The model under review builds one solid part; all positions refer to its coordinate system, in mm. A direction names the side the tool comes from. Round coordinates to 2 decimals unless told otherwise and drop trailing zeros. Order: outer loops, then holes, each group sorted by start corner. A loop starts at its lowest first (then second) coordinate and runs counter-clockwise, first axis right, second up. Notation, with made-up numbers: M 48,-11 L 100,-11 A20 ccw 100,27 Z; hole C 6.5,-12 d4. An arc over 180 degrees is marked long. Answer as a JSON object with one key per item and string values. Group by question number.
1) For faces 1 (the flat face through (30.94, -1, 2)), 2 (the flat face through (2, 11.298, 2)), 3 (the cylindrical face through (54.597, 7.345, 1.551)), 4 (the flat face through (25.06, 46, 2)), list the 3-axis set-ups (+Z, -Z, +X, -X, +Y, -Y) from which the entire face can be reached by the end or side of a thin tool; tool diameter is ignored.
2) Consider section A-A, the plane x = 2.5. Write out the cut boundary in (y, z), then the cut area to 3 significant figures.
3) To check wall thickness, follow line 1 (Y direction, x = 53.5, z = 0.85); line 2 (Y direction, x = 2.5, z = 2.3); line 3 (X direction, y = 26.5, z = 0.95). State the ranges of each line that lie inside material, in increasing order.
4) Consider section B-B, the plane z = 1.5. Write out the cut boundary in (x, y).
5) Consider section D-D, the plane y = 20.5. Write out the cut boundary in (x, z).
6) Consider section C-C, the plane x = 53.5. Write out the cut boundary in (y, z).
7) Insertion check: pin 1 Ø0.9 at (x, z) = (27, 1.5) entering from -Y. The pin has a flat end and moves straight along its axis. Give the tip position at first contact, or say it passes through.
8) The part is to be moulded in two halves that separate along X. For faces 5 (the flat face through (0, 41, 2)), 6 (the flat face through (13, 48, 2)), 7 (the cylindrical face through (2.251, 36.377, 1.551)), say which applies: +X half, -X half, draft (parallel to the pull), parting line (faces both ways), or undercut.
```python
from build123d import *

# Parameters (mm, degrees)
BOSS_EXTRUDE1_DEPTH = 3.06
SKETCH2_R           = 1.15
SKETCH2_W           = 4
SKETCH2_H           = 22.201866978
CUT_EXTRUDE1_DEPTH  = 74.819804931


with BuildPart() as part:
    # Sketch1 → Boss-Extrude1 (new body)
    with BuildSketch(Plane.XY):
        Polygon((25.06, 0), (30.94, 0), (30.94, -3), (56, -3), (56, 0), (56, 45), (56, 48), (30.94, 48), (30.94, 45), (25.06, 45), (25.06, 48), (0, 48), (0, 45), (0, 0), (0, -3), (25.06, -3), align=None)
    extrude(amount=BOSS_EXTRUDE1_DEPTH)

    # Sketch2 → Cut-Extrude1 (cut, through all)
    with BuildSketch(Plane.XY.offset(3.06)):
        with Locations((2.5, 37.5)):
            Circle(SKETCH2_R)
        with Locations((53.5, 37.5)):
            Circle(SKETCH2_R)
        with Locations((53.5, 7)):
            Circle(SKETCH2_R)
        with Locations((2.5, 7)):
            Circle(SKETCH2_R)
        with Locations((2, 22.399066511)):
            Rectangle(SKETCH2_W, SKETCH2_H)
    extrude(amount=-CUT_EXTRUDE1_DEPTH, mode=Mode.SUBTRACT)


solid = part.part
```
Results list:
{
 "1": {"face 1": "+Z, -Z, -Y", "face 2": "+Z, -Z, -X", "face 3": "+Z, -Z", "face 4": "+Z, -Z, +Y"},
 "2": {"outline": "M -3,0 L 5.85,0 L 5.85,3.06 L -3,3.06 Z; M 8.15,0 L 11.3,0 L 11.3,3.06 L 8.15,3.06 Z; M 33.5,0 L 36.35,0 L 36.35,3.06 L 33.5,3.06 Z; M 38.65,0 L 48,0 L 48,3.06 L 38.65,3.06 Z", "area": "74.0 mm^2"},
 "3": {"line 1": "-3 to 5.85, 8.15 to 36.35, 38.65 to 48", "line 2": "-3 to 5.85, 8.15 to 11.3, 33.5 to 36.35, 38.65 to 48", "line 3": "4 to 56"},
 "4": {"outline": "M 0,-3 L 25.06,-3 L 25.06,0 L 30.94,0 L 30.94,-3 L 56,-3 L 56,48 L 30.94,48 L 30.94,45 L 25.06,45 L 25.06,48 L 0,48 L 0,33.5 L 4,33.5 L 4,11.3 L 0,11.3 Z; hole C 2.5,7 d2.3; hole C 2.5,37.5 d2.3; hole C 53.5,7 d2.3; hole C 53.5,37.5 d2.3"},
 "5": {"outline": "M 4,0 L 56,0 L 56,3.06 L 4,3.06 Z"},
 "6": {"outline": "M -3,0 L 5.85,0 L 5.85,3.06 L -3,3.06 Z; M 8.15,0 L 36.35,0 L 36.35,3.06 L 8.15,3.06 Z; M 38.65,0 L 48,0 L 48,3.06 L 38.65,3.06 Z"},
 "7": {"pin 1": "y = 0"},
 "8": {"face 5": "-X half", "face 6": "draft", "face 7": "undercut"}
}
